from build123d import *

# Parameters (mm, degrees)
SKETCH1_W            = 29.7
SKETCH1_H            = 67
BOSS_EXTRUDE1_DEPTH  = 6
SKETCH2_R            = 1.5
CUT_EXTRUDE1_DEPTH   = 87
SKETCH3_W            = 42
SKETCH3_H            = 6
BOSS_EXTRUDE2_DEPTH  = 58
SKETCH4_W            = 14
SKETCH4_H            = 9
CUT_EXTRUDE2_DEPTH   = 58
SKETCH8_W            = 5
SKETCH8_H            = 58
BOSS_EXTRUDE5_DEPTH  = 6
BOSS_EXTRUDE3_DEPTH  = 0.5
BOSS_EXTRUDE4_DEPTH  = 5
FILLET1_R            = 1
FILLET1_OF_MIRROR1_R = 1
SKETCH7_R            = 4
CUT_EXTRUDE3_DEPTH   = 1


with BuildPart() as part:
    # Sketch1 → Boss-Extrude1 (new body)
    with BuildSketch(Plane.XY):
        Rectangle(SKETCH1_W, SKETCH1_H)
    extrude(amount=BOSS_EXTRUDE1_DEPTH)

    # Sketch2 → Cut-Extrude1 (cut)
    with BuildSketch(Plane(origin=(14.85, 0, 0), x_dir=(0, 0, -1), z_dir=(1, 0, 0))):
        with Locations((-3, -29.5)):
            Circle(SKETCH2_R)
    extrude(amount=-CUT_EXTRUDE1_DEPTH, mode=Mode.SUBTRACT)

    # Sketch3 → Boss-Extrude2 (add)
    with BuildSketch(Plane(origin=(0, 33.5, 0), x_dir=(1, 0, 0), z_dir=(0, 1, 0))):
        with Locations((0, -3)):
            Rectangle(SKETCH3_W, SKETCH3_H)
    extrude(amount=-BOSS_EXTRUDE2_DEPTH)

    # Sketch4 → Cut-Extrude2 (cut)
    with BuildSketch(Plane(origin=(0, 0, 0), x_dir=(-1, 0, 0), z_dir=(0, 0, -1))):
        with Locations((0, -29)):
            Rectangle(SKETCH4_W, SKETCH4_H)
    extrude(amount=-CUT_EXTRUDE2_DEPTH, mode=Mode.SUBTRACT)

    # Sketch8 → Boss-Extrude5 (add)
    with BuildSketch(Plane.XY.offset(6)):
        with Locations((-23.5, 4.5)):
            Rectangle(SKETCH8_W, SKETCH8_H)
        with Locations((23.5, 4.5)):
            Rectangle(SKETCH8_W, SKETCH8_H)
    extrude(amount=-BOSS_EXTRUDE5_DEPTH)

    # Sketch5 → Boss-Extrude3 (add)
    with BuildSketch(Plane(origin=(0, 0, 0), x_dir=(-1, 0, 0), z_dir=(0, 0, -1))):
        Polygon((26, -24.5), (26, 33.5), (-26, 33.5), (-26, -24.5), (-14.85, -24.5), (-14.85, -33.5), (-7, -33.5), (-7, -24.5), (7, -24.5), (7, -33.5), (14.85, -33.5), (14.85, -24.5), align=None)
    extrude(amount=BOSS_EXTRUDE3_DEPTH)

    # Sketch6 → Boss-Extrude4 (add)
    with BuildSketch(Plane(origin=(0, 0, -0.5), x_dir=(-1, 0, 0), z_dir=(0, 0, -1))):
        Polygon((-22, 29.5), (-22, -18.5), (-18, -18.5), (-18, 25.5), (-2, 25.5), (-2, 29.5), align=None)
    boss_extrude4 = extrude(amount=BOSS_EXTRUDE4_DEPTH)

    # Fillet1
    fillet1_edges = [part.edges().sort_by_distance(p)[0] for p in [
        (12, 29.5, -5.5),
        (22, 5.5, -5.5),
        (20, -18.5, -5.5),
        (18, 3.5, -5.5),
        (10, 25.5, -5.5),
        (2, 27.5, -5.5),
    ]]
    fillet(fillet1_edges, radius=FILLET1_R)

    # Mirror1: Boss-Extrude4 across plane
    add(boss_extrude4.mirror(Plane(origin=(0, 0, 0), x_dir=(0, 0, 1), z_dir=(1, 0, 0))))

    # Fillet1 of Mirror1
    fillet1_of_mirror1_edges = [part.edges().sort_by_distance(p)[0] for p in [
        (-12, 29.5, -5.5),
        (-22, 5.5, -5.5),
        (-20, -18.5, -5.5),
        (-18, 3.5, -5.5),
        (-10, 25.5, -5.5),
        (-2, 27.5, -5.5),
    ]]
    fillet(fillet1_of_mirror1_edges, radius=FILLET1_OF_MIRROR1_R)

    # Sketch7 → Cut-Extrude3 (cut)
    with BuildSketch(Plane.XY.offset(6)):
        with Locations((0, 20.200252003)):
            Circle(SKETCH7_R)
    extrude(amount=-CUT_EXTRUDE3_DEPTH, mode=Mode.SUBTRACT)


solid = part.part
Verification items for the finished model (mm, model axes). A direction names the side the tool comes from. Round coordinates to 2 decimals unless told otherwise and drop trailing zeros. Loops run counter-clockwise (first coordinate to the right, second up) from the corner with the lowest first, then second, coordinate; pieces in that order, holes last. Notation, with made-up numbers: M 86,6 L 143,6 A30 cw 143,34 Z; hole C 82,64 d2. An arc over 180 degrees is marked long. Write each question's results on one line, items separated by ' | '.
1) Section check D-D on z = 3. Record the boundary of the cut face in (x, y).
Checks:
outline: M -26,-24.5 L -14.85,-24.5 L -14.85,-28 L -7,-28 L -7,-24.5 L 7,-24.5 L 7,-28 L 14.85,-28 L 14.85,-24.5 L 26,-24.5 L 26,33.5 L -26,33.5 Z; M -14.85,-33.5 L -7,-33.5 L -7,-31 L -14.85,-31 Z; M 7,-33.5 L 14.85,-33.5 L 14.85,-31 L 7,-31 Z
2) Scan lines: L1, parallel to Y at x = 0, z = 5.3; L2, parallel to Y at x = 9.75, z = 3; L3, parallel to X at y = -26.5, z = 3.75. Record each from-to range of solid material in increasing order. Write a range as from..to.
Checks:
L1: y = -24.5..16.2, 24.2..33.5 | L2: y = -33.5..-31, -28..33.5 | L3: x = -14.85..-7, 7..14.85
3) Mould release check, pull along X, two halves, no side actions. Record for faces 1 (the flat face through (11, -33.5, 3)), 2 (the flat face through (7, -28, 2)), 3 (the cylindrical face through (-0.521, 24.166, 5.507)), 4 (the flat face through (22, 6, -2)): released by +X, released by -X, zero draft, split by the parting line, or undercut.
Checks:
face 1: zero draft | face 2: undercut | face 3: undercut | face 4: released by +X
4) Gauge pin test, flat ends, axial feed: P1, Ø1.2, axis at x = 19.5, z = -2.5, coming from the -Y side; P2, Ø4.5, axis at x = -20.5, z = -1.5, coming from the -Y side; P3, Ø1.2, axis at y = 11, z = -3, coming from the -X side; P4, Ø4.5, axis at y = -3.5, z = -2, coming from the +X side. Record the tip position at first contact, or that the pin passes through.
Checks:
P1: stops at y = -18.5 | P2: stops at y = -24.5 | P3: stops at x = -22 | P4: stops at x = 26
5) Section check C-C on x = 11. Record the boundary of the cut face in (y, z).
Checks:
outline: M -33.5,-0.5 L 25.5,-0.5 L 25.5,-4.5 A1 ccw 26.5,-5.5 L 28.5,-5.5 A1 ccw 29.5,-4.5 L 29.5,-0.5 L 33.5,-0.5 L 33.5,6 L -33.5,6 Z; hole C -29.5,3 d3
6) Access from +Z, -Z, +X, -X, +Y, -Y to the whole of each face (thin tool, end or side, straight path). Record for faces 5 (the flat face through (-14.85, -28, 2)), 6 (the flat face through (21, -24.5, 3)), 7 (the flat face through (20, -18.5, -2)).
Checks:
face 5: +Z, -Z, -X, -Y | face 6: +Z, -Z, +X, -Y | face 7: -Z, +X, -X, -Y
7) Section check A-A on z = -2. Record the boundary of the cut face in (x, y).
Checks:
outline: M -22,-18.5 L -18,-18.5 L -18,25.5 L -2,25.5 L -2,29.5 L -22,29.5 Z; M 2,25.5 L 18,25.5 L 18,-18.5 L 22,-18.5 L 22,29.5 L 2,29.5 Z
8) Section check B-B on y = -29.5. Record the boundary of the cut face in (x, z).
Checks:
outline: M -14.85,-0.5 L -7,-0.5 L -7,1.5 L -14.85,1.5 Z; M -14.85,4.5 L -7,4.5 L -7,6 L -14.85,6 Z; M 7,-0.5 L 14.85,-0.5 L 14.85,1.5 L 7,1.5 Z; M 7,4.5 L 14.85,4.5 L 14.85,6 L 7,6 Z
